Geometry: final body of the model. Coordinates: model frame, mm. A direction names the side the tool comes from. Give positions to 0.01 mm unless a question says otherwise; leave off trailing zeros. Loops run counter-clockwise (first coordinate to the right, second up) from the corner with the lowest first, then second, coordinate; pieces in that order, holes last.
from build123d import *

# Parameters (mm, degrees)
F0_R     = 10.6194281647
F1_DEPTH = 33.274
F3_R     = 5.08
F4_T     = -2.54
F5_DEPTH = 19.558


# Not quite as in the source:
# - the program builds the solid bodies; features that only make, move or delete a surface that nothing else refers to are left out


with BuildPart() as f1:
    # F0 (on Front) → F1 (new body)
    with BuildSketch(Plane.XZ):
        Polygon((0, 17.026649788), (-64.4087642431, 54.5603483915), (-67.7721425891, -4.5970836654), align=None)
        with Locations((-48.2645332813, 22.2235824913)):
            Circle(F0_R, mode=Mode.SUBTRACT)
        with Locations((-48.2645332813, 22.2235824913)):
            Circle(F0_R)
    extrude(amount=F1_DEPTH)

    # F3
    f3_edges = [f1.edges().sort_by_distance(p)[0] for p in [
        (-33.886071, 0, 6.214783),
        (-32.204382, 0, 35.793499),
        (-66.090453, 0, 24.981632),
    ]]
    fillet(f3_edges, radius=F3_R)

    # F4
    f4_openings = [f1.faces().sort_by_distance(p)[0] for p in [
        (-44.060302, -33.274, 22.329972),
    ]]
    offset(amount=F4_T, openings=f4_openings)

    # F5 (add): a face of the model
    f5_faces = [f1.faces().sort_by_distance(p)[0] for p in [
        (-32.2043821216, -19.177, 35.7934990898),
    ]]
    extrude(f5_faces, amount=F5_DEPTH)


solid = f1.part
Item 1: Set-up query: faces 1 (the face through (-34.36, -18.98, 6.063)), 2 (the face through (-27, -5.08, 44)), 3 (the face through (-35.43, -3.3, 9.15)). Return all of +Z, -Z, +X, -X, +Y, -Y with unobstructed straight access to the full face (end or side cutting, diameter ignored); none if empty.
Values follow:
face 1: -Z, +X, +Y, -Y
face 2: +Z, +X, +Y
face 3: -Y
Item 2: Section query A-A on y = -14. Return loops of the section in (x, z), plus the area to 3 significant figures.
Values follow:
outline: (-67.77, -4.6) - (0, 17.03) - (9.85, 33.92) - (-54.56, 71.46) - (-64.41, 54.56) - close; hole (-65.03, -1.05) - (-6.22, 17.71) - (-62.11, 50.28) - close
area: 1,940 mm2
Item 3: Draft query along X for faces 4 (the face through (-21.91, -18.98, 52.43)), 5 (the face through (-64.67, -1.53, 24.49)), 6 (the face through (-43, -2.54, 25)), 7 (the face through (-32, -33.274, 35)). Return one class per face: +X half, -X half, draft (parallel to the pull), parting line (faces both ways), or undercut.
Values follow:
face 4: +X half
face 5: -X half
face 6: undercut
face 7: draft
Item 4: Ray query, probe 1 along Y at (x, z) = (-28.5, 37); probe 2 along X at (y, z) = (-4, 36); probe 3 along Z at (x, y) = (-55.5, -28). Return the intervals inside material, ascending.
Values follow:
probe 1: y = -33.27 to -5.08
probe 2: x = -65.35 to -62.68, -38.08 to -32.79
probe 3: z = -0.68 to 1.98, 46.43 to 69.85
Item 5: Section query B-B on z = 57.5. Return loops of the section in (x, y).
Values follow:
outline: (-62.7, -33.27) - (-30.61, -33.27) - (-30.61, -5.08) - (-62.7, -5.08) - close
Item 6: Section query C-C on y = -4. Return loops of the section in (x, z).
Values follow:
outline: (-67.65, -4.44) - (-0.28, 17.06) - (-64.3, 54.36) - close; hole (-64.77, -0.72) - (-6.81, 17.77) - (-61.89, 49.87) - close
Item 7: Pin query (flat end, axial travel): pin 1 (6 mm diameter, centred on x = -59.5, y = -26, fed in from -Z); pin 2 (1.5 mm diameter, centred on y = -10.5, z = 57, fed in from +X); pin 3 (6 mm diameter, centred on x = -54, y = -7, fed in from -Z). Return the tip coordinate at first contact, or that it passes through.
Values follow:
pin 1: stops at z = -2.91
pin 2: stops at x = -28.46
pin 3: stops at z = -1.16
